Check sheet for the modelled part. Datum: model origin and axes. Units: mm. A direction names the side the tool comes from. Round coordinates to 2 decimals unless told otherwise and drop trailing zeros. Order: outer loops, then holes, each group sorted by start corner. A loop starts at its lowest first (then second) coordinate and runs counter-clockwise, first axis right, second up.
Autodesk Inventor part; units mm, degrees
ref_plane "YZ Plane" through (0, 0, 0) normal (1, 0, 0) x (0, 1, 0)
ref_plane "XZ Plane" through (0, 0, 0) normal (0, 1, 0) x (-1, 0, 0)
ref_plane "XY Plane" through (0, 0, 0) normal (0, 0, 1) x (1, 0, 0)
sketch "Sketch1" plane through (0, 0, 0) normal (0, 0, 1) x (1, 0, 0)
  line L0 (0, 0) -> (38.1, 0)
  line L1 (38.1, 0) -> (38.1, 3.175)
  line L2 (38.1, 3.175) -> (0, 3.175)
  line L3 (0, 3.175) -> (0, 0)
  dimension "d0" = 38.1
  dimension "d1" = 3.175
extrude "Extrusion1" add sketch "Sketch1" along normal blind 355.6
sketch "Sketch2" plane through (0, 0, 355.6) normal (0, 0, 1) x (1, 0, 0)
  line L0 (0, 0) -> (3.175, 0)
  line L1 (3.175, 0) -> (3.175, 38.1)
  line L2 (3.175, 38.1) -> (0, 38.1)
  line L3 (0, 38.1) -> (0, 0)
  dimension "d4" = 3.175
  dimension "d5" = 38.1
extrude "Extrusion2" add sketch "Sketch2" against normal blind 355.6
properties part number "14in L Channel"
1) Gauge pin test, flat end, axial feed: pin 1 (4 mm diameter, centred on x = 12, z = 212, fed in from +Y) (3 decimals). Record the tip position at first contact, or that the pin passes through.
2) Set-up check for faces 1 (the face through (0, 19, 175)), 2 (the face through (21, 3.175, 175)): record each of +Z, -Z, +X, -X, +Y, -Y from which the full face is reachable in a straight line by a thin tool's end or side.
3) Sectioned sample at A-A on z = 71. Record the cut outline in (x, y) (3 decimals), and give its area (3 significant figures).
4) Scan line: line 1 (Y direction, x = 19, z = 177) (3 decimals). Record every from-to range of solid material in increasing order.
5) Sectioned sample at B-B on y = 20. Record the cut outline in (x, z) (3 decimals), and give its area (3 significant figures).
Values found:
1. pin 1: stops at y = 3.175
2. face 1: +Z, -Z, -X, +Y, -Y
2. face 2: +Z, -Z, +X, +Y
3. outline: (0, 0) - (38.1, 0) - (38.1, 3.175) - (3.175, 3.175) - (3.175, 38.1) - (0, 38.1) - close
3. area: 232 mm2
4. line 1: y = 0 to 3.175
5. outline: (0, 0) - (3.175, 0) - (3.175, 355.6) - (0, 355.6) - close
5. area: 1,130 mm2
